Geometry check sheet. Reference: the model listing, model coordinates, mm. Give positions to 0.01 mm unless a question says otherwise; leave off trailing zeros. Write each loop counter-clockwise with the first axis right and the second up, starting at its lowest first coordinate (ties: lowest second). Pieces come first, ordered by that corner, then holes. Notation, with made-up numbers: (-30, -1) - (19, -1) arc R24 cw to (19, 9) - close; hole circle Ø8 at (17, 49.25). An arc over 180 degrees is marked (long way). One line per question, with ' | ' between items. Start each with the question number.
Q1. Gauge pin test, flat end, axial feed: P1, Ø22.5, axis at x = -73.025, y = 85.725, coming from the +Z side (3 decimals). Record the tip position at first contact, or that the pin passes through.
Q2. Thickness scan on L1, parallel to X at y = 85.5, z = 1; L2, parallel to X at y = 84, z = -2; L3, parallel to X at y = 30, z = 0.75. Record the ranges inside material, lowest first. Write a range as [from, to].
Q3. Section check C-C on z = -1.75. Record the boundary of the cut face in (x, y) (3 decimals), and give its area (3 significant figures).
Q4. Section check B-B on x = -72. Record the boundary of the cut face in (y, z) (3 decimals).
Q5. Section check D-D on x = 70.5. Record the boundary of the cut face in (y, z) (3 decimals).
Q6. Section check A-A on y = 88.5. Record the boundary of the cut face in (x, z) (3 decimals), and give its area (3 significant figures).
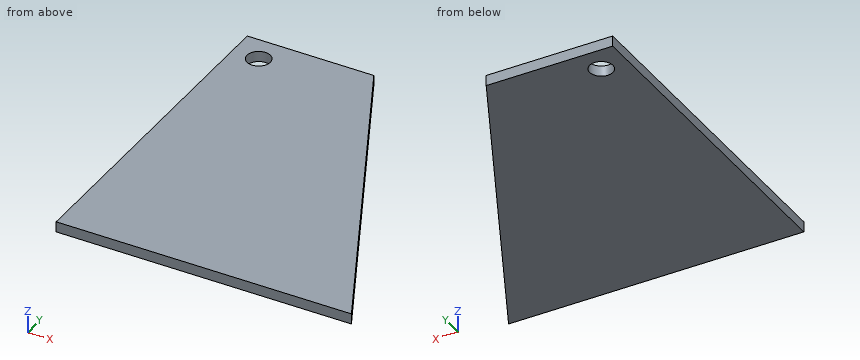
```python
from build123d import *

# Parameters (mm, degrees)
SKETCH1_R           = 6.985
BOSS_EXTRUDE1_DEPTH = 3.175


with BuildPart() as part:
    # Sketch1 → Boss-Extrude1 (new body, symmetric)
    with BuildSketch(Plane.XY):
        Polygon((-88.9, 101.6), (-88.9, -101.6), (88.9, -101.6), (-12.7, 101.6), align=None)
        with Locations((-73.025, 85.725)):
            Circle(SKETCH1_R, mode=Mode.SUBTRACT)
    extrude(amount=BOSS_EXTRUDE1_DEPTH, both=True)


solid = part.part
```
Working result:
1) P1: stops at z = 3.175
2) L1: x = [-88.9, -80.01], [-66.04, -4.65] | L2: x = [-88.9, -79.79], [-66.26, -3.9] | L3: x = [-88.9, 23.1]
3) outline: (-88.9, -101.6) - (88.9, -101.6) - (-12.7, 101.6) - (-88.9, 101.6) - close; hole circle Ø13.97 at (-73.025, 85.725) | area: 25,700 mm2
4) outline: (-101.6, -3.175) - (78.816, -3.175) - (78.816, 3.175) - (-101.6, 3.175) - close; (92.634, -3.175) - (101.6, -3.175) - (101.6, 3.175) - (92.634, 3.175) - close
5) outline: (-101.6, -3.175) - (-64.8, -3.175) - (-64.8, 3.175) - (-101.6, 3.175) - close
6) outline: (-88.9, -3.175) - (-79.435, -3.175) - (-79.435, 3.175) - (-88.9, 3.175) - close; (-66.615, -3.175) - (-6.15, -3.175) - (-6.15, 3.175) - (-66.615, 3.175) - close | area: 444 mm2
